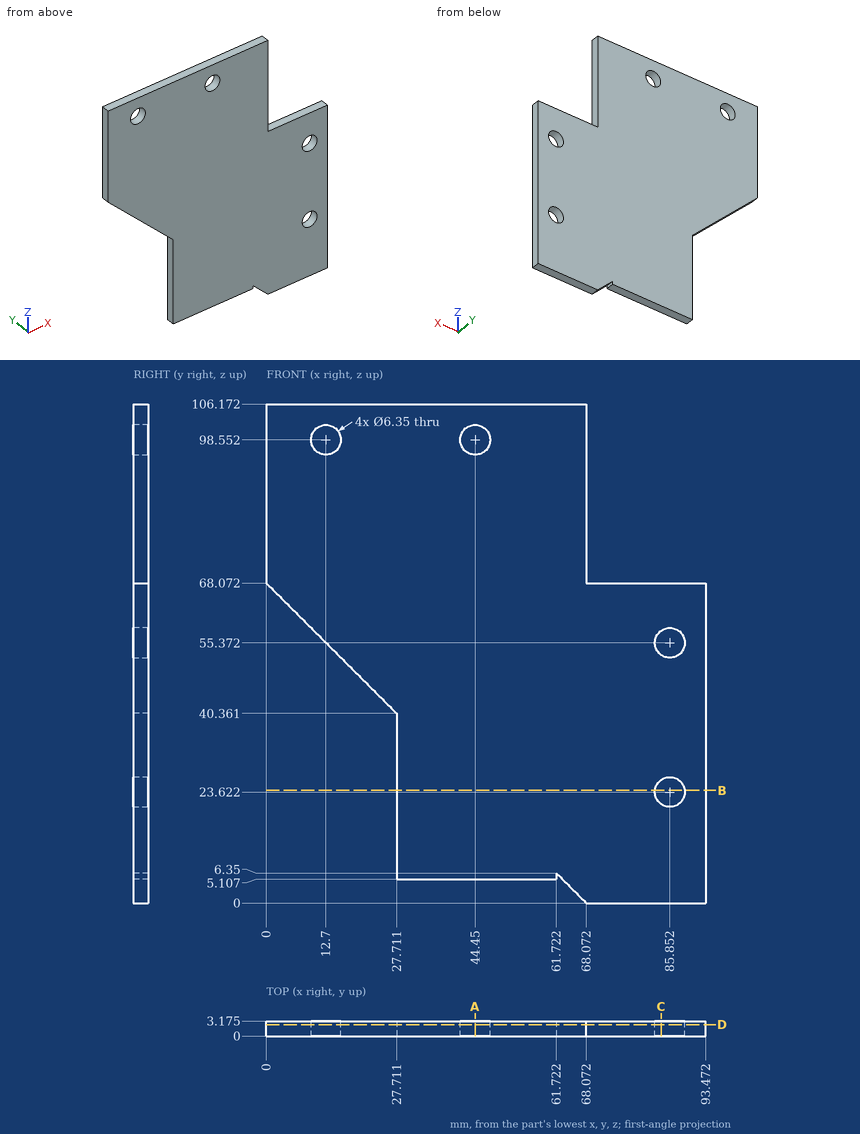
Geometry: see drawing. Coordinates: mm, zero at the bounding-box minimum. Round coordinates to 2 decimals unless told otherwise and drop trailing zeros. Write each loop counter-clockwise with the first axis right and the second up, starting at its lowest first coordinate (ties: lowest second). Pieces come first, ordered by that corner, then holes. Notation, with made-up numbers: (38.25, 64.25) - (47.25, 64.25) arc R14 cw to (47.25, 87.25) - close; hole circle Ø2 at (86.5, -23). An arc over 180 degrees is marked (long way). Use CSV: the item, a comma, the result in double quotes. Start each with the question number.
(1) Material intervals for probe 1 along X at (y, z) = (0.4, 73); probe 2 along Z at (x, y) = (30, 0.9), sorted ascending. Write a range as [from, to].
(2) Cut plane A-A, the plane x = 44.45. Return loops of the section in (y, z) (1 decimal).
(3) Cut plane D-D, the plane y = 2.4. Give the number of separate pieces and of enclosed holes in the cut face, and give its area (3 significant figures).
(4) Cut plane C-C, the plane x = 84. Return loops of the section in (y, z) (1 decimal).
(5) Cut plane B-B, the plane z = 24. Return loops of the section in (x, y) (1 decimal), and give its area (3 significant figures).
(6) First-contact query: pin 1 Ø3 at (x, z) = (14, 65.5) entering from -Y; pin 2 Ø1 at (x, y) = (71, 1) entering from +Z; pin 3 Ø1 at (y, z) = (2, 21) entering from -X; pin 4 Ø1 at (y, z) = (1.5, 85.5) entering from +X. Flat tips, straight axial feed; report the tip coordinate or a pass-through.
Geometry says:
1,probe 1,"[0, 68.07]"
1,probe 2,"[5.11, 106.17]"
2,outline,"(0, 5.1) - (3.2, 5.1) - (3.2, 95.4) - (0, 95.4) - close; (0, 101.7) - (3.2, 101.7) - (3.2, 106.2) - (0, 106.2) - close"
3,separate pieces,"1"
3,enclosed holes,"4"
3,area,"7,130 mm²"
4,outline,"(0, 0) - (3.2, 0) - (3.2, 21) - (0, 21) - close; (0, 26.2) - (3.2, 26.2) - (3.2, 52.8) - (0, 52.8) - close; (0, 58) - (3.2, 58) - (3.2, 68.1) - (0, 68.1) - close"
5,outline,"(27.7, 0) - (82.7, 0) - (82.7, 3.2) - (27.7, 3.2) - close; (89, 0) - (93.5, 0) - (93.5, 3.2) - (89, 3.2) - close"
5,area,"189 mm²"
6,pin 1,"y = 0"
6,pin 2,"z = 68.07"
6,pin 3,"x = 27.71"
6,pin 4,"x = 68.07"
